Source: CAD feature listing. Evaluate the final solid. Frame: model axes, mm. A direction names the side the tool comes from. Give positions to 0.01 mm unless a question says otherwise; leave off trailing zeros. Order: outer loops, then holes, each group sorted by start corner. A loop starts at its lowest first (then second) coordinate and runs counter-clockwise, first axis right, second up. Notation, with made-up numbers: M -14,-0.5 L 36,-0.5 A29 cw 36,28.5 Z; hole C 68.25,5 d10. An arc over 180 degrees is marked long. Answer in a Markdown table with one row per item. Add a question column.
(1) Section query C-C, the plane x = -63.5. Return loops of the section in (y, z), plus the area to 3 significant figures.
(2) Set-up query: faces 1 (the face through (-70.327, 36.109, -12.522)), 2 (the face through (-120.561, 25.958, 177.788)), 3 (the face through (-12.7, 26, 113)). Return all of +Z, -Z, +X, -X, +Y, -Y with unobstructed straight access to the full face (end or side cutting, diameter ignored); none if empty.
(3) Material intervals for line 1 along Y through (x, z) = (-120.25, 165.1); line 2 along X through (y, z) = (49.5, 82.5); line 3 along Z through (x, y) = (-117, 25), sorted ascending.
(4) Pin query (flat end, axial travel): P1, Ø23, axis at y = 25.4, z = 165.1, coming from the -X side; P2, Ø5, axis at x = -13, y = 18, coming from the -Z side; P3, Ø3, axis at x = -52, y = 32.5, coming from the +Z side. Return the tip coordinate at first contact, or that it passes through.
(5) Mould query, pull axis Y, two halves, no side actions, for faces 4 (the face through (-116, 0, 79)), 5 (the face through (-6.261, 25.958, 177.788)), 6 (the face through (-114.3, 26, 116)), 7 (the face through (-64, 50.8, 23)). Classes: pulls with the +Y half, pulls with the -Y half, needs draft (parallel to the pull), parting line crosses it, or undercut.
(6) Section query B-B, the plane z = 165.1. Return loops of the section in (x, y), plus the area to 3 significant figures.
(7) Section query A-A, the plane z = 53. Return loops of the section in (x, y).
(8) Section query D-D, the plane y = 31. Return loops of the section in (x, z), plus the area to 3 significant figures.
from build123d import *

# Parameters (mm, degrees)
SKETCH1_W           = 127
SKETCH1_H           = 203.2
BOSS_EXTRUDE1_DEPTH = 50.8
CUT_EXTRUDE1_DEPTH  = 254
SKETCH4_R           = 12.7
CUT_EXTRUDE2_DEPTH  = 254
SKETCH5_R           = 12.7
BOSS_EXTRUDE2_DEPTH = 25.4
FILLET1_R           = 25.4
FILLET2_R           = 25.4


with BuildPart() as part:
    # Sketch1 → Boss-Extrude1 (new body)
    with BuildSketch(Plane(origin=(0, 0, 0), x_dir=(1, 0, 0), z_dir=(0, 1, 0))):
        with Locations((-63.5, -101.6)):
            Rectangle(SKETCH1_W, SKETCH1_H)
    extrude(amount=BOSS_EXTRUDE1_DEPTH)

    # Sketch3 → Cut-Extrude1 (cut)
    with BuildSketch(Plane(origin=(0, 50.8, 0), x_dir=(1, 0, 0), z_dir=(0, 1, 0))):
        Polygon((-63.5, -25.4), (-12.7, -25.4), (-12.7, -203.2), (-114.3, -203.2), (-114.3, -25.4), align=None)
    extrude(amount=-CUT_EXTRUDE1_DEPTH, mode=Mode.SUBTRACT)

    # Sketch4 → Cut-Extrude2 (cut)
    with BuildSketch(Plane(origin=(0, 0, 0), x_dir=(0, 0, -1), z_dir=(1, 0, 0))):
        with Locations((-165.1, 25.4)):
            Circle(SKETCH4_R)
    extrude(amount=-CUT_EXTRUDE2_DEPTH, mode=Mode.SUBTRACT)

    # Sketch5 → Boss-Extrude2 (add)
    with BuildSketch(Plane(origin=(0, 0, 0), x_dir=(-1, 0, 0), z_dir=(0, 0, -1))):
        with Locations((63.5, 25.4)):
            Circle(SKETCH5_R)
    extrude(amount=BOSS_EXTRUDE2_DEPTH)

    # Fillet1
    fillet1_edges = [part.edges().sort_by_distance(p)[0] for p in [
        (-120.65, 50.8, 203.2),
    ]]
    fillet(fillet1_edges, radius=FILLET1_R)

    # Fillet2
    fillet2_edges = [part.edges().sort_by_distance(p)[0] for p in [
        (-6.35, 50.8, 203.2),
    ]]
    fillet(fillet2_edges, radius=FILLET2_R)


solid = part.part
Values follow:
| question | item | result |
|---|---|---|
| 1 | outline | M 0,0 L 12.7,0 L 12.7,-25.4 L 38.1,-25.4 L 38.1,0 L 50.8,0 L 50.8,25.4 L 0,25.4 Z |
| 1 | area | 1,940 mm² |
| 2 | face 1 | -Z |
| 2 | face 2 | +X, -X |
| 2 | face 3 | +Z, +Y, -Y |
| 3 | line 1 | y = 0 to 12.7, 38.1 to 50.8 |
| 3 | line 2 | x = -127 to -114.3, -12.7 to 0 |
| 3 | line 3 | z = 0 to 152.41, 177.79 to 203.2 |
| 4 | P1 | passes through |
| 4 | P2 | stops at z = 0 |
| 4 | P3 | stops at z = 25.4 |
| 5 | face 4 | pulls with the -Y half |
| 5 | face 5 | undercut |
| 5 | face 6 | needs draft |
| 5 | face 7 | pulls with the +Y half |
| 6 | outline | M -127,0 L -114.3,0 L -114.3,12.7 L -127,12.7 Z; M -127,38.1 L -114.3,38.1 L -114.3,50.8 L -127,50.8 Z; M -12.7,0 L 0,0 L 0,12.7 L -12.7,12.7 Z; M -12.7,38.1 L 0,38.1 L 0,50.8 L -12.7,50.8 Z |
| 6 | area | 645 mm² |
| 7 | outline | M -127,0 L -114.3,0 L -114.3,50.8 L -127,50.8 Z; M -12.7,0 L 0,0 L 0,50.8 L -12.7,50.8 Z |
| 8 | outline | M -127,0 L -74.9,0 L -74.9,-25.4 L -52.1,-25.4 L -52.1,0 L 0,0 L 0,153.7 L -12.7,153.7 L -12.7,25.4 L -114.3,25.4 L -114.3,153.7 L -127,153.7 Z; M -127,176.5 L -114.3,176.5 L -114.3,202.57 L -127,202.57 Z; M -12.7,176.5 L 0,176.5 L 0,202.57 L -12.7,202.57 Z |
| 8 | area | 7,730 mm² |
